Geometry check sheet. Reference: the model listing, model coordinates, mm. A direction names the side the tool comes from. Round coordinates to 2 decimals unless told otherwise and drop trailing zeros. Loops run counter-clockwise (first coordinate to the right, second up) from the corner with the lowest first, then second, coordinate; pieces in that order, holes last.
```python
from build123d import *

# Parameters (mm, degrees)
CHAMFER1_SIZE = 0.25


with BuildPart() as part:
    # Sketch1 → Revolve1 (revolve)
    with BuildSketch(Plane.XY):
        Polygon((2, 0), (2, 1), (5, 4), (10.5, 4), (10.5, 38), (12.5, 38), (12.5, 0), align=None)
    revolve(axis=Axis((0, -587.15114798, 0), (0, 1, 0)))

    # Chamfer1
    chamfer1_edges = [part.edges().sort_by_distance(p)[0] for p in [
        (-12.5, 0, 0),
        (-12.5, 38, 0),
        (-10.5, 38, 0),
        (-2, 0, 0),
    ]]
    chamfer(chamfer1_edges, length=CHAMFER1_SIZE)


solid = part.part
```
1) Scan lines: line 1 along Z through (x, y) = (0, 0.6); line 2 along Z through (x, y) = (0, 30.5). Record each from-to range of solid material in increasing order.
Report:
line 1: z = -12.5 to -2, 2 to 12.5
line 2: z = -12.5 to -10.5, 10.5 to 12.5
2) Gauge pin test, flat ends, axial feed: pin 1 (1 mm diameter, centred on y = 4.5, z = 6.5, fed in from +X); pin 2 (5 mm diameter, centred on x = 8, y = 7, fed in from +Z) (3 decimals); pin 3 (3.5 mm diameter, centred on x = 0, z = 0, fed in from +Y); pin 4 (8 mm diameter, centred on x = 3, z = -1, fed in from +Y). Record the tip position at first contact, or that the pin passes through.
Report:
pin 1: stops at x = 10.97
pin 2: stops at z = 11.225
pin 3: passes through
pin 4: stops at y = 4
3) Sectioned sample at C-C, the plane y = 13. Record the cut outline in (x, z), then the cut area to 3 significant figures.
Report:
outline: circle Ø25 at (0, 0); hole circle Ø21 at (0, 0)
area: 145 mm2
4) Sectioned sample at A-A, the plane z = 0. Record the cut outline in (x, y).
Report:
outline: (-12.5, 0.25) - (-12.25, 0) - (-2.25, 0) - (-2, 0.25) - (-2, 1) - (-5, 4) - (-10.5, 4) - (-10.5, 37.75) - (-10.75, 38) - (-12.25, 38) - (-12.5, 37.75) - close; (2, 0.25) - (2.25, 0) - (12.25, 0) - (12.5, 0.25) - (12.5, 37.75) - (12.25, 38) - (10.75, 38) - (10.5, 37.75) - (10.5, 4) - (5, 4) - (2, 1) - close
5) Mould release check, pull along X, two halves, no side actions. Record for faces 3 (the face through (11.923, 18.738, -3.755)), 4 (the face through (-0.434, 0.63, 1.952)), 5 (the face through (3, 0, 0)): +X half, -X half, draft (parallel to the pull), parting line (faces both ways), or undercut.
Report:
face 3: parting line
face 4: undercut
face 5: draft
6) Sectioned sample at B-B, the plane x = 0. Record the cut outline in (y, z), then the cut area to 3 significant figures.
Report:
outline: (0, -12.25) - (0.25, -12.5) - (37.75, -12.5) - (38, -12.25) - (38, -10.75) - (37.75, -10.5) - (4, -10.5) - (4, -5) - (1, -2) - (0.25, -2) - (0, -2.25) - close; (0, 2.25) - (0.25, 2) - (1, 2) - (4, 5) - (4, 10.5) - (37.75, 10.5) - (38, 10.75) - (38, 12.25) - (37.75, 12.5) - (0.25, 12.5) - (0, 12.25) - close
area: 211 mm2
7) Access from +Z, -Z, +X, -X, +Y, -Y to the whole of each face (thin tool, end or side, straight path). Record for faces 1 (the face through (0, 38, 11)), 2 (the face through (-5, 4, 2)).
Report:
face 1: +Z, -Z, +X, -X, +Y
face 2: +Y
